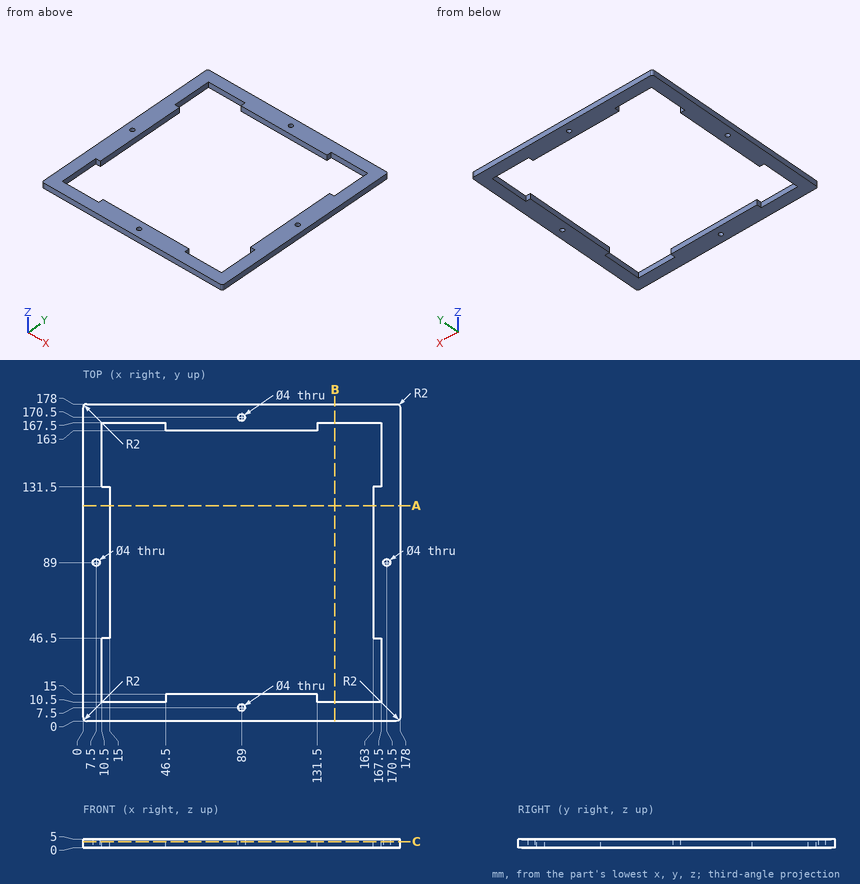
Check sheet for the drawn part. Datum: minimum x, y, z corner. Units: mm. Round coordinates to 2 decimals unless told otherwise and drop trailing zeros. Write each loop counter-clockwise with the first axis right and the second up, starting at its lowest first coordinate (ties: lowest second). Pieces come first, ordered by that corner, then holes. Notation, with made-up numbers: (-9.75, 67.5) - (39.25, 67.5) arc R21 cw to (39.25, 93.5) - close; hole circle Ø9 at (69, 16.5). An arc over 180 degrees is marked (long way). Write each question's results on one line, items separated by ' | '.
(1) Thickness scan on probe 1 along X at (y, z) = (89, 1.6); probe 2 along Y at (x, z) = (142, 2.15). Record the ranges inside material, lowest first. Write a range as from..to.
Computed:
probe 1: x = 0..5.5, 9.5..15, 163..168.5, 172.5..178 | probe 2: y = 0..10.5, 167.5..178
(2) Sectioned sample at C-C, the plane z = 3.55. Count the separate pieces of the cut face and the enclosed holes in it, plus the area to 3 significant figures.
Computed:
separate pieces: 1 | enclosed holes: 5 | area: 8,510 mm^2
(3) Sectioned sample at A-A, the plane y = 121. Enter the section's corners in (x, z).
Computed:
outline: (0, 0) - (15, 0) - (15, 5) - (0, 5) - close; (163, 0) - (178, 0) - (178, 5) - (163, 5) - close
(4) Sectioned sample at B-B, the plane x = 141.5. Enter the section's corners in (y, z), plus the area to 3 significant figures.
Computed:
outline: (0, 0) - (10.5, 0) - (10.5, 5) - (0, 5) - close; (167.5, 0) - (178, 0) - (178, 5) - (167.5, 5) - close | area: 105 mm^2
